The model under review builds one solid part; all positions refer to its coordinate system, in mm. A direction names the side the tool comes from. Coordinates: 2 decimals unless noted, no trailing zeros. Write each loop counter-clockwise with the first axis right and the second up, starting at its lowest first coordinate (ties: lowest second). Pieces come first, ordered by that corner, then holes.
1) Mouldability with a two-part tool opening along Z and no side actions: class faces 1 (the flat face through (6, 1, 7.358)), 2 (the flat face through (9.901, 1, 1)), 3 (the flat face through (-10, 1, 2.568)), 4 (the flat face through (3.981, 1, 1)) as released by +Z, released by -Z, zero draft, split by the parting line, or undercut.
2) For P1, Ø4, axis at x = 6, z = 7.5, coming from the +Y side; P2, Ø0.9, axis at x = 6.5, y = 2, coming from the +Z side; P3, Ø0.9, axis at y = 2, z = 8.5, coming from the +X side; P4, Ø0.9, axis at x = 7.5, y = 1.5, coming from the -Z side, all flat-tipped, find the tip position at first contact; note any pin that passes through.
3) Add section B-B, the plane y = 1.2. State the section outline as (x, z) points, then the cut area to 3 significant figures.
4) For line 1 (X direction, y = 0.65, z = 2.5); line 2 (Z direction, x = 6.75, y = 0.7); line 3 (Z direction, x = 8, y = 1.35), list the stretches that pass through material, from the lowest coordinate up.
5) Add section A-A, the plane x = 6.5. State the section outline as (y, z) points, then the cut area to 3 significant figures.
6) Machinability: for faces 5 (the flat face through (2.901, 1, -7)), 6 (the flat face through (2.901, 1, 9)), 7 (the flat face through (-7.099, 1, -7)), 8 (the flat face through (-10, 1, -0.352)), which of the approach directions +Z, -Z, +X, -X, +Y, -Y give a long, thin tool a straight path to every point of the face, cutting with its end or side? Answer none if there is none.
from build123d import *

# Parameters (mm, degrees)
SKETCH1_W           = 10
SKETCH1_H           = 3
BOSS_EXTRUDE1_DEPTH = 3


with BuildPart() as part:
    # Sketch1 → Boss-Extrude1 (new body)
    with BuildSketch(Plane(origin=(0, 0, 0), x_dir=(1, 0, 0), z_dir=(0, 1, 0))):
        with BuildLine():
            Line((9.900990099, -7.357973937), (9.900990099, -1.107973937))
            Line((9.900990099, -1.107973937), (6.900990099, -1.107973937))
            Line((6.900990099, -1.107973937), (6.900990099, -2.567973937))
            Line((6.900990099, -2.567973937), (3.980990099, -2.567973937))
            Line((3.980990099, -2.567973937), (3.980990099, -1.107973937))
            Line((3.980990099, -1.107973937), (-1.099009901, -1.107973937))
            ThreePointArc((-1.099009901, -1.107973937), (-2.099009901, -2.107973937), (-3.099009901, -1.107973937))
            Line((-3.099009901, -1.107973937), (-8.179009901, -1.107973937))
            Line((-8.179009901, -1.107973937), (-8.179009901, -2.567973937))
            Line((-8.179009901, -2.567973937), (-11.099009901, -2.567973937))
            Line((-11.099009901, -2.567973937), (-11.099009901, -1.107973937))
            Line((-11.099009901, -1.107973937), (-14.099009901, -1.107973937))
            Line((-14.099009901, -1.107973937), (-14.099009901, -7.357973937))
            Line((-14.099009901, -7.357973937), (-7.099009901, -7.357973937))
            Line((-7.099009901, -7.357973937), (2.900990099, -7.357973937))
            Line((2.900990099, -7.357973937), (9.900990099, -7.357973937))
        make_face()
        with BuildLine():
            Line((9.900990099, 5.142026063), (2.900990099, 5.142026063))
            Line((2.900990099, 5.142026063), (-7.099009901, 5.142026063))
            Line((-7.099009901, 5.142026063), (-14.099009901, 5.142026063))
            Line((-14.099009901, 5.142026063), (-14.099009901, -1.107973937))
            Line((-14.099009901, -1.107973937), (-11.099009901, -1.107973937))
            Line((-11.099009901, -1.107973937), (-11.099009901, 0.352026063))
            Line((-11.099009901, 0.352026063), (-8.179009901, 0.352026063))
            Line((-8.179009901, 0.352026063), (-8.179009901, -1.107973937))
            Line((-8.179009901, -1.107973937), (-3.099009901, -1.107973937))
            ThreePointArc((-3.099009901, -1.107973937), (-2.099009901, -0.107973937), (-1.099009901, -1.107973937))
            Line((-1.099009901, -1.107973937), (3.980990099, -1.107973937))
            Line((3.980990099, -1.107973937), (3.980990099, 0.352026063))
            Line((3.980990099, 0.352026063), (6.900990099, 0.352026063))
            Line((6.900990099, 0.352026063), (6.900990099, -1.107973937))
            Line((6.900990099, -1.107973937), (9.900990099, -1.107973937))
            Line((9.900990099, -1.107973937), (9.900990099, 5.142026063))
        make_face()
        with Locations((-2.099009901, 6.642026063)):
            Rectangle(SKETCH1_W, SKETCH1_H)
        with Locations((-2.099009901, -8.857973937)):
            Rectangle(SKETCH1_W, SKETCH1_H)
    extrude(amount=BOSS_EXTRUDE1_DEPTH)


solid = part.part
Geometry results:
1. face 1: released by +Z
1. face 2: zero draft
1. face 3: undercut
1. face 4: undercut
2. P1: stops at y = 3
2. P2: stops at z = 7.36
2. P3: stops at x = 2.9
2. P4: stops at z = -5.14
3. outline: (-14.1, -5.14) - (-7.1, -5.14) - (-7.1, -8.14) - (2.9, -8.14) - (2.9, -5.14) - (9.9, -5.14) - (9.9, 7.36) - (2.9, 7.36) - (2.9, 10.36) - (-7.1, 10.36) - (-7.1, 7.36) - (-14.1, 7.36) - close; hole (-11.1, -0.35) - (-8.18, -0.35) - (-8.18, 2.57) - (-11.1, 2.57) - close; hole circle Ø2 at (-2.1, 1.11); hole (3.98, -0.35) - (6.9, -0.35) - (6.9, 2.57) - (3.98, 2.57) - close
3. area: 340 mm2
4. line 1: x = -14.1 to -11.1, -8.18 to 3.98, 6.9 to 9.9
4. line 2: z = -5.14 to -0.35, 2.57 to 7.36
4. line 3: z = -5.14 to 7.36
5. outline: (0, -5.14) - (3, -5.14) - (3, -0.35) - (0, -0.35) - close; (0, 2.57) - (3, 2.57) - (3, 7.36) - (0, 7.36) - close
5. area: 28.7 mm2
6. face 5: -Z, +X, +Y, -Y
6. face 6: +Z, +X, +Y, -Y
6. face 7: -Z, -X, +Y, -Y
6. face 8: +Y, -Y
